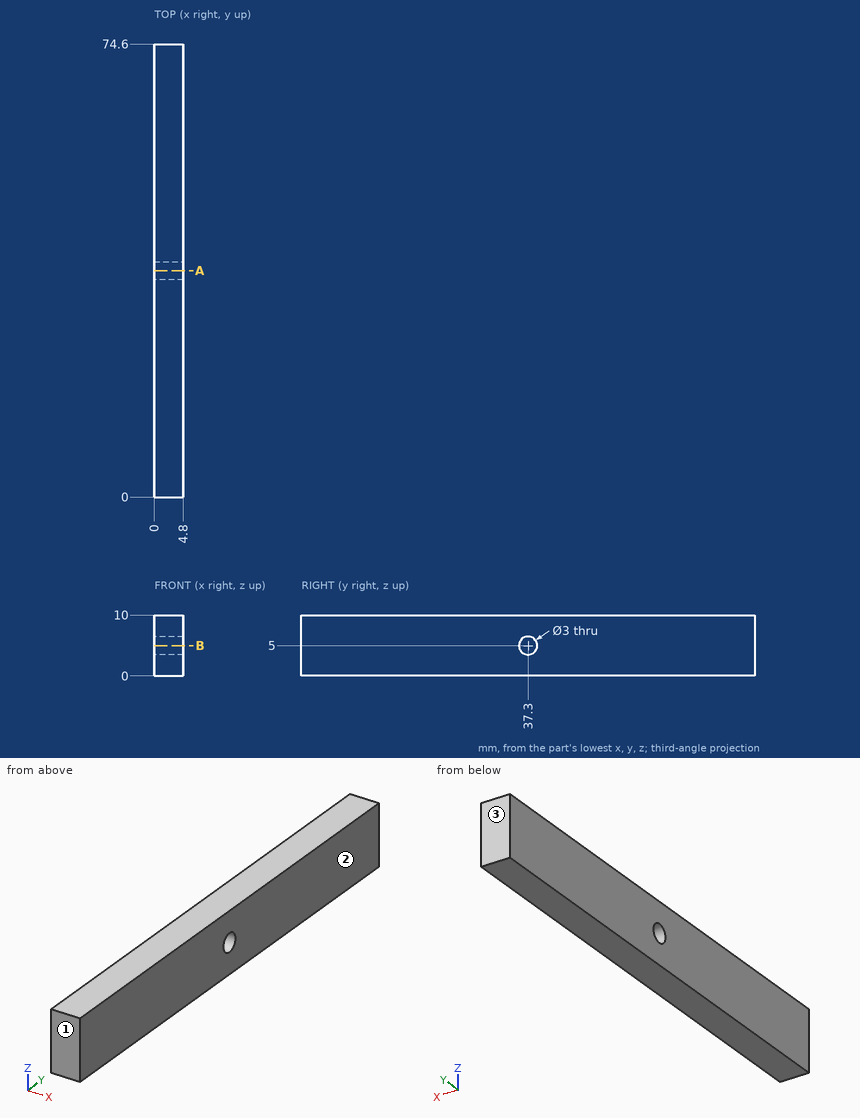
Source: three-view drawing plus pictorial views. Frame: mm from the lowest corner of the part. Round coordinates to 2 decimals unless told otherwise and drop trailing zeros. Write each loop counter-clockwise with the first axis right and the second up, starting at its lowest first coordinate (ties: lowest second). Pieces come first, ordered by that corner, then holes. Notation, with made-up numbers: M -2.5,11.25 L 45.5,11.25 A13 ccw 45.5,24.25 Z; hole C 24.5,89 d10. An arc over 180 degrees is marked long. Write each question's results on one line, items separated by ' | '.
Q1. Draft query along Y for the marked faces 1, 2 and 3. Return one class per face: released by +Y, released by -Y, zero draft, split by the parting line, or undercut.
Results:
face 1: released by -Y | face 2: zero draft | face 3: released by +Y
Q2. Section query A-A (y = 37.3). Return loops of the section in (x, z), and give its area (3 significant figures).
Results:
outline: M 0,0 L 4.8,0 L 4.8,3.5 L 0,3.5 Z; M 0,6.5 L 4.8,6.5 L 4.8,10 L 0,10 Z | area: 33.6 mm^2
Q3. Line query: line 1 along Z through (x, y) = (1.2, 37.3); line 2 along Z through (x, y) = (2.15, 36). Output: solid intervals per line, ascending.
Results:
line 1: z = 0 to 3.5, 6.5 to 10 | line 2: z = 0 to 4.25, 5.75 to 10
Q4. Section query B-B (z = 5). Return loops of the section in (x, y).
Results:
outline: M 0,0 L 4.8,0 L 4.8,35.8 L 0,35.8 Z; M 0,38.8 L 4.8,38.8 L 4.8,74.6 L 0,74.6 Z
